from build123d import *

# Parameters (mm, degrees)
F0_W     = 203.2
F0_H     = 127
F1_DEPTH = 127
F3_DEPTH = 76.2
F4_SIZE2 = 101.6
F4_SIZE  = 76.2
F5_R     = 5.08
F6_R     = 15.24
F7_DEPTH = 50.8
F8_R     = 19.349676851
F9_DEPTH = 127


with BuildPart() as f1:
    # F0 (on Front) → F1 (new body)
    with BuildSketch(Plane.XZ):
        with Locations((38.9206162602, 27.6787289854)):
            Rectangle(F0_W, F0_H)
    extrude(amount=F1_DEPTH)

    # F2 (on face) → F3 (cut)
    with BuildSketch(Plane.XZ.offset(127)):
        Polygon((38.9206162602, 27.6787289854), (0.8206162602, 27.6787289854), (0.8206162602, -35.8212710146), (140.5206162602, -35.8212710146), (140.5206162602, 91.1787289854), (38.9206162602, 91.1787289854), align=None)
    extrude(amount=-F3_DEPTH, mode=Mode.SUBTRACT)

    # F4
    f4_edges = [f1.edges().sort_by_distance(p)[0] for p in [
        (140.520616, -25.4, 91.178729),
    ]]
    f4_side = f1.faces().sort_by_distance((17.149188, -52.614286, 91.178729))[0]
    chamfer(f4_edges, length=F4_SIZE, length2=F4_SIZE2, reference=f4_side)

    # F5
    f5_edges = [f1.edges().sort_by_distance(p)[0] for p in [
        (-11.879384, -127, 91.178729),
        (38.920616, -127, 59.428729),
        (19.870616, -127, 27.678729),
        (0.820616, -127, -4.071271),
        (38.920616, -88.9, 27.678729),
        (-62.679384, -127, 27.678729),
        (0.820616, -88.9, 27.678729),
        (0.820616, -88.9, -35.821271),
        (0.820616, -50.8, -4.071271),
        (38.920616, -50.8, 59.428729),
        (38.920616, -88.9, 91.178729),
        (0.820616, 0, 91.178729),
        (64.320616, -25.4, 91.178729),
        (-62.679384, -63.5, 91.178729),
        (51.620616, -50.8, 91.178729),
        (-30.929384, -127, -35.821271),
        (70.670616, -50.8, -35.821271),
        (19.870616, -50.8, 27.678729),
    ]]
    fillet(f5_edges, radius=F5_R)

    # F6 (on face) → F7 (cut, through all)
    with BuildSketch(Plane.XZ.offset(50.8)):
        with Locations((56.7006162602, 0)):
            Circle(F6_R)
    extrude(amount=-F7_DEPTH, mode=Mode.SUBTRACT)

    # F8 (on face) → F9 (cut, through all)
    with BuildSketch(Plane.XY.offset(91.1787289854)):
        with Locations((-25.0357538462, -37.260428071)):
            Circle(F8_R)
    extrude(amount=-F9_DEPTH, mode=Mode.SUBTRACT)


solid = f1.part
The listing builds one solid part. Answer for the finished solid, in the listing's coordinates (mm). A direction names the side the tool comes from. Round coordinates to 2 decimals unless told otherwise and drop trailing zeros. Order: outer loops, then holes, each group sorted by start corner. A loop starts at its lowest first (then second) coordinate and runs counter-clockwise, first axis right, second up. Notation, with made-up numbers: (50, 41) - (67, 41) arc R21 cw to (67, 57) - close; hole circle Ø6 at (49.5, 33.5). An arc over 180 degrees is marked (long way). Write item = value, one per line. Start each with the question number.
1) For faces 5 (the cylindrical face through (37.393, -88.438, 89.73)), 6 (the flat face through (15, 0, 26)), 7 (the flat face through (72, -50.8, 16)), determine the directions among +Z, -Z, +X, -X, +Y, -Y from which every point of the face is accessible in a straight line to the end or side of a thin tool.
2) Section C-C, the plane x = -28 is taken. Write down the section's boundary in (y, z), plus the area to 3 significant figures.
3) Given pin 1 (1.5 mm diameter, centred on x = 72.5, z = 29.5, fed in from -Y); pin 2 (8 mm diameter, centred on x = 0, z = -6.5, fed in from -Y); pin 3 (8 mm diameter, centred on y = -18, z = 67, fed in from +X), each flat-ended and moving along its own axis, determine where each tip first touches the part or whether it passes through.
4) For a pull along X with two mould halves and no side action, classify faces 1 (the cylindrical face through (70.779, -25.756, -5.837)), 2 (the cylindrical face through (-61.231, -125.472, 25.992)), 3 (the cylindrical face through (-33.06, -125.551, -34.294)), 4 (the flat face through (140.521, -25, -23)) as released by +X, released by -X, zero draft, split by the parting line, or undercut.
5) Straight lines are drawn through the part: L1, parallel to X at y = -45, z = -11; L2, parallel to X at y = -116, z = -9; L3, parallel to Y at x = 54.5, z = 31. For each, find the intervals that lie inside material, in ascending order.
6) Section B-B, the plane z = 11 is taken. Write down the section's boundary in (x, y).
7) Section A-A, the plane y = -21 is taken. Write down the section's boundary in (x, z).
8) Section D-D, the plane y = -107 is taken. Write down the section's boundary in (x, z), plus the area to 3 significant figures.
Results list:
q1.face_5 = +Z, +X, -Y
q1.face_6 = +Z, -Z, +X, -X, +Y
q1.face_7 = -Z, +X, -Y
q2.outline = (-127, -30.74) arc R5.08 ccw to (-121.92, -35.82) - (-56.38, -35.82) - (-56.38, 91.18) - (-121.92, 91.18) arc R5.08 ccw to (-127, 86.1) - close; (-18.14, -35.82) - (0, -35.82) - (0, 86.1) arc R5.08 ccw to (-5.08, 91.18) - (-18.14, 91.18) - close
q2.area = 11,300 mm^2
q3.pin_1 = -50.8
q3.pin_2 = -126.99
q3.pin_3 = 85.45
q4.face_1 = undercut
q4.face_2 = released by -X
q4.face_3 = zero draft
q4.face_4 = released by +X
q5.L1 = -62.68 to -42.77, -7.3 to 46.15, 67.25 to 140.52
q5.L2 = -62.68 to 0.82
q5.L3 = -50.8 to 0
q6.outline = (-62.68, -121.92) arc R5.08 ccw to (-57.6, -127) - (-4.26, -127) arc R5.08 ccw to (0.82, -121.92) - (0.82, -55.88) arc R5.08 cw to (5.9, -50.8) - (46.15, -50.8) - (46.15, 0) - (-62.68, 0) - close; (67.25, -50.8) - (124.45, -50.8) - (124.45, 0) - (67.25, 0) - close; hole circle Ø38.7 at (-25.04, -37.26)
q7.outline = (-62.68, -35.82) - (-35.52, -35.82) - (-35.52, 91.18) - (-57.6, 91.18) arc R5.08 ccw to (-62.68, 86.1) - close; (-14.55, -35.82) - (140.52, -35.82) - (140.52, -10.42) - (65.84, 89.15) arc R5.08 ccw to (61.78, 91.18) - (-14.55, 91.18) - close; hole circle Ø30.48 at (56.7, 0)
q8.outline = (-62.68, -35.82) - (-4.26, -35.82) arc R5.08 ccw to (0.82, -30.74) - (0.82, 22.6) arc R5.08 cw to (5.9, 27.68) - (33.84, 27.68) arc R5.08 ccw to (38.92, 32.76) - (38.92, 86.1) arc R5.08 ccw to (33.84, 91.18) - (-57.6, 91.18) arc R5.08 ccw to (-62.68, 86.1) - close
q8.area = 10,500 mm^2
